from build123d import *

# Parameters (mm, degrees)
F0_W     = 114.3
F0_H     = 50.8
F1_DEPTH = 3.175
F2_DEPTH = 152.4
F4_DEPTH = 3.302
F5_R     = 15.24
F6_R     = 12.7
F7_DEPTH = 3.175
F8_SIZE  = 3.17499


# Not quite as in the source:
# - a fillet or chamfer is up to 0.001 mm smaller than in the source, because OpenCascade refuses the exact size


with BuildPart() as f1:
    # F0 (on Top) → F1 (new body)
    with BuildSketch(Plane.XY):
        Rectangle(F0_W, F0_H)
    extrude(amount=F1_DEPTH)

    # F2 (add): a face of the model
    f2_faces = [f1.faces().sort_by_distance(p)[0] for p in [
        (0, 25.4, 1.5875),
    ]]
    extrude(f2_faces, amount=F2_DEPTH)

    # F3 (on face) → F4 (cut)
    with BuildSketch(Plane.XY.offset(3.175)):
        Polygon((-13.97, 155.8029547439), (13.97, 155.8029547439), (26.67, 177.8), (-26.67, 177.8), align=None)
    extrude(amount=-F4_DEPTH, mode=Mode.SUBTRACT)

    # F5
    f5_edges = [f1.edges().sort_by_distance(p)[0] for p in [
        (13.97, 155.802955, 1.5875),
        (-13.97, 155.802955, 1.5875),
    ]]
    fillet(f5_edges, radius=F5_R)

    # F6
    f6_edges = [f1.edges().sort_by_distance(p)[0] for p in [
        (57.15, -25.4, 1.5875),
        (-57.15, -25.4, 1.5875),
    ]]
    fillet(f6_edges, radius=F6_R)

    # F3 (on face) → F7 (cut)
    with BuildSketch(Plane.XY.offset(3.175)):
        Polygon((57.15, 76.2), (57.15, 119.1976362049), (41.91, 110.3988181024), (41.91, 84.9988181024), align=None)
        Polygon((-41.91, 110.3988181024), (-57.15, 119.1976362049), (-57.15, 76.2), (-41.91, 84.9988181024), align=None)
    extrude(amount=-F7_DEPTH, mode=Mode.SUBTRACT)

    # F8 (size 3.175 in the source; OpenCascade refuses exactly that, so slightly less here)
    f8_edges = [f1.edges().sort_by_distance(p)[0] for p in [
        (-22.519705, 170.611477, 3.175),
        (-12.791182, 157.844728, 3.175),
        (0, 155.802955, 3.175),
        (12.791182, 157.844728, 3.175),
        (22.519705, 170.611477, 3.175),
    ]]
    chamfer(f8_edges, length=F8_SIZE)


solid = f1.part
Input: part model. Units: mm. Frame: model coordinates. A direction names the side the tool comes from. Round coordinates to 2 decimals unless told otherwise and drop trailing zeros. Write each loop counter-clockwise with the first axis right and the second up, starting at its lowest first coordinate (ties: lowest second). Pieces come first, ordered by that corner, then holes.
1) Cut plane C-C (y = 98). Return the cut outline in (x, z) (3 decimals), then the cut area to 3 significant figures.
2) Ray query, L1, parallel to X at y = 106, z = 2.95; L2, parallel to X at y = 157, z = 0.8; L3, parallel to Y at x = -8, z = 1.95. Return the intervals inside material, ascending.
3) Draft query along Y for faces 1 (the conical face through (13.315, 156.696, 1.257)), 2 (the flat face through (-49.637, 80.538, 1.61)), 3 (the flat face through (-1, 75, 3.175)). Return one class per face: pulls with the +Y half, pulls with the -Y half, needs draft (parallel to the pull), parting line crosses it, or undercut.
4) Reachability of faces 4 (the flat face through (-49.423, 114.737, 1.61)), 5 (the conical face through (-13.524, 156.817, 1.257)), 6 (the flat face through (49.64, 114.86, 1.61)) from +Z, -Z, +X, -X, +Y, -Y: full face, straight path, thin tool, end or side. Return the list, or none.
5) Cut plane B-B (z = 1.3). Return the cut outline in (x, y), then the cut area to 3 significant figures.
6) Contact query for flat-ended pins moving along their axis: P1, Ø12, axis at x = 19.5, y = 133, coming from the -Z side; P2, Ø1, axis at y = 100.5, z = 2, coming from the +X side. Output: stop coordinate, or through.
Geometry says:
1. outline: (-41.91, 0) - (41.91, 0) - (41.91, 3.175) - (-41.91, 3.175) - close
1. area: 266 mm2
2. L1: x = -41.91 to 41.91
2. L2: x = -57.15 to -12.92, 12.92 to 57.15
2. L3: y = -25.4 to 154.09
3. face 1: pulls with the +Y half
3. face 2: undercut
3. face 3: needs draft
4. face 4: +Z, -Z, -X
4. face 5: +Z, +Y
4. face 6: +Z, -Z, +X
5. outline: (-57.15, -12.7) arc R12.7 ccw to (-44.45, -25.4) - (44.45, -25.4) arc R12.7 ccw to (57.15, -12.7) - (57.15, 76.2) - (41.91, 85) - (41.91, 110.4) - (57.15, 119.2) - (57.15, 177.8) - (28.17, 177.8) - (19.5, 162.77) arc R16.54 cw to (5.17, 154.5) - (-5.17, 154.5) arc R16.54 cw to (-19.5, 162.77) - (-28.17, 177.8) - (-57.15, 177.8) - (-57.15, 119.2) - (-41.91, 110.4) - (-41.91, 85) - (-57.15, 76.2) - close
5. area: 21,100 mm2
6. P1: stops at z = 0
6. P2: stops at x = 41.91
